Geometry: see drawing. Coordinates: mm, zero at the bounding-box minimum. A direction names the side the tool comes from. Coordinates: 2 decimals unless noted, no trailing zeros. Loops run counter-clockwise (first coordinate to the right, second up) from the corner with the lowest first, then second, coordinate; pieces in that order, holes last. Notation, with made-up numbers: (70, -18.5) - (114, -18.5) arc R22 ccw to (114, 1.5) - close; hole circle Ø1 at (33, 6). An arc over 180 degrees is marked (long way). Answer in a Markdown table with one row per item.
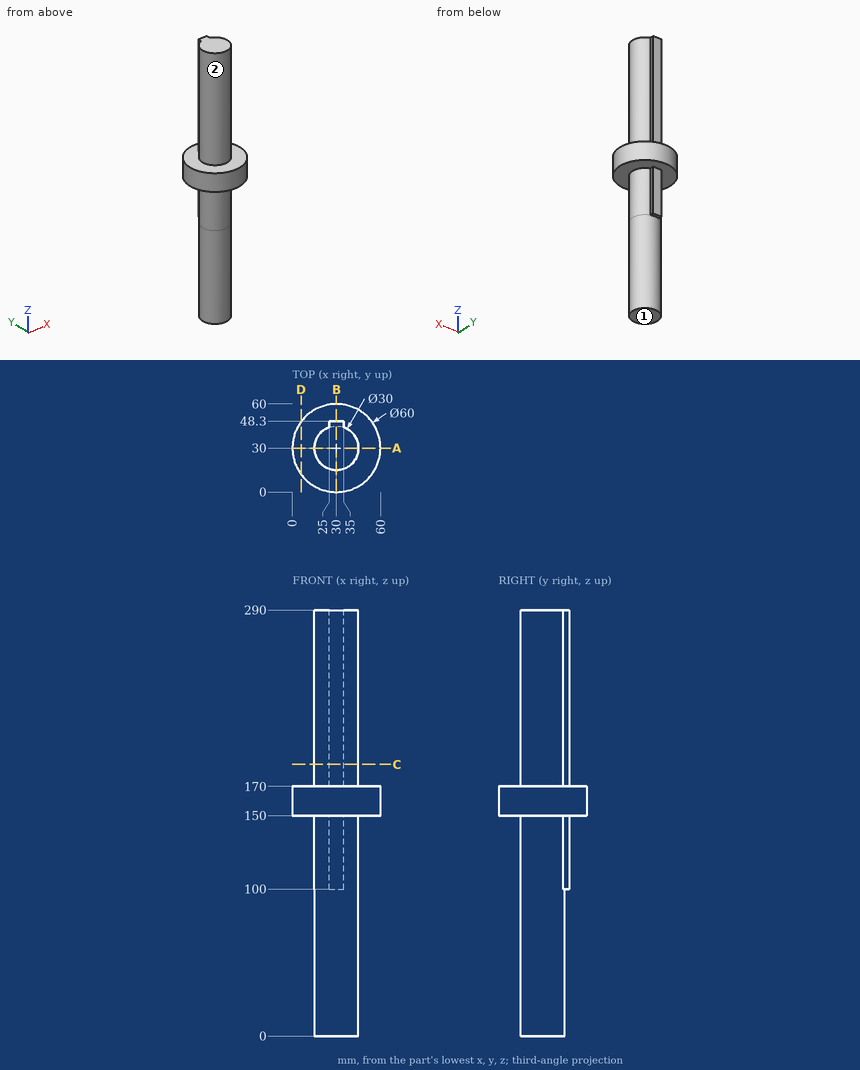
(1) Cut plane A-A on y = 30. Output: boundary loops of the cut face in (x, z).
Verdict:
| item | result |
|---|---|
| outline | (0, 150) - (15, 150) - (15, 0) - (45, 0) - (45, 150) - (60, 150) - (60, 170) - (45, 170) - (45, 290) - (15, 290) - (15, 170) - (0, 170) - close |
(2) First-contact query: pin 1 Ø6 at (x, z) = (46.5, 244.5) entering from -Y; pin 2 Ø3.5 at (y, z) = (46.5, 116) entering from -X; pin 3 Ø8 at (x, z) = (34.5, 65) entering from +Y. Flat tips, straight axial feed; report the tip coordinate or a pass-through.
Verdict:
| item | result |
|---|---|
| pin 1 | stops at y = 23.46 |
| pin 2 | stops at x = 25 |
| pin 3 | stops at y = 44.99 |
(3) Cut plane C-C on z = 185. Output: boundary loops of the cut face in (x, y).
Verdict:
| item | result |
|---|---|
| outline | (25, 44.14) arc R15 ccw (long way) to (35, 44.14) - (35, 48.3) - (25, 48.3) - close |
(4) Cut plane B-B on x = 30. Output: boundary loops of the cut face in (y, z).
Verdict:
| item | result |
|---|---|
| outline | (0, 150) - (15, 150) - (15, 0) - (45, 0) - (45, 100) - (48.3, 100) - (48.3, 150) - (60, 150) - (60, 170) - (48.3, 170) - (48.3, 290) - (15, 290) - (15, 170) - (0, 170) - close |
(5) Cut plane D-D on x = 6. Output: boundary loops of the cut face in (y, z).
Verdict:
| item | result |
|---|---|
| outline | (12, 150) - (48, 150) - (48, 170) - (12, 170) - close |
(6) Access query for the marked faces 1 and 2. Directions: +Z, -Z, +X, -X, +Y, -Y. A direction counts if a zero-diameter tool reaches every point of the face in a straight line with its end or side. Return the directions, or none.
Verdict:
| item | result |
|---|---|
| face 1 | -Z, +X, -X, +Y, -Y |
| face 2 | +Z |
(7) Ray query, probe 1 along Z at (x, y) = (44.5, 17); probe 2 along X at (y, z) = (35.5, 256); probe 3 along X at (y, z) = (25, 273). Return the intervals inside material, ascending.
Verdict:
| item | result |
|---|---|
| probe 1 | z = 150 to 170 |
| probe 2 | x = 16.04 to 43.96 |
| probe 3 | x = 15.86 to 44.14 |
